Check sheet for the modelled part. Datum: model origin and axes. Units: mm. A direction names the side the tool comes from. Give positions to 0.01 mm unless a question says otherwise; leave off trailing zeros. Order: outer loops, then holes, each group sorted by start corner. A loop starts at its lowest first (then second) coordinate and runs counter-clockwise, first axis right, second up. Notation, with made-up numbers: (69, 36.5) -> (103, 36.5) arc R28 cw to (103, 59.5) -> close; hole circle Ø1 at (-8, 44). An arc over 180 degrees is marked (long way). One line per question, with ' | ' between items.
```python
from build123d import *

# Parameters (mm, degrees)
F1_DEPTH = 15
F3_DEPTH = 25
F4_R     = 3.99999
F5_W     = 7.0163438655
F5_H     = 17.1485144225
F6_DEPTH = 25
F7_R     = 2.6
F8_R     = 2.8
F9_DEPTH = 25
F10_R    = 20
F11_R    = 4


# Not quite as in the source:
# - a fillet or chamfer is up to 0.001 mm smaller than in the source, because OpenCascade refuses the exact size


with BuildPart() as f1:
    # F0 (on Right) → F1 (new body)
    with BuildSketch(Plane.YZ):
        Polygon((-44.9859467229, 8), (-66.9859467229, 8), (-66.9859467229, 0), (-44.9859467229, 0), (41.0894067598, -30.7737162478), (42.3002508738, -27.5966470596), (43.3758810707, -24.7743584453), (44.6834651639, -21.3434583933), align=None)
    extrude(amount=F1_DEPTH)

    # F2 (on face) → F3 (cut)
    with BuildSketch(Plane(origin=(0, 0, 0), x_dir=(1, 0, 0), z_dir=(0, 0, -1))):
        with BuildLine():
            Line((4.5, 58.9859467229), (4.5, 52.9859467229))
            ThreePointArc((4.5, 52.9859467229), (7.5, 49.9859467229), (10.5, 52.9859467229))
            Line((10.5, 52.9859467229), (10.5, 58.9859467229))
            ThreePointArc((10.5, 58.9859467229), (7.5, 61.9859467229), (4.5, 58.9859467229))
        make_face()
    extrude(amount=-F3_DEPTH, mode=Mode.SUBTRACT)

    # F4 (radius 4 in the source; OpenCascade refuses exactly that, so slightly less here)
    f4_edges = [f1.edges().sort_by_distance(p)[0] for p in [
        (7.5, -66.985947, 0),
        (7.5, -66.985947, 8),
    ]]
    fillet(f4_edges, radius=F4_R)

    # F5 (on face) → F6 (cut)
    with BuildSketch(Plane(origin=(0, -1.9867064016, -6.0710906068), x_dir=(1, 0, 0), z_dir=(0, 0.3110113487, 0.9504061979))):
        with Locations((11.4918280672, 40.5312428041)):
            Rectangle(F5_W, F5_H)
        Polygon((15, 49.1055000154), (15, 31.9569855928), (21.9836561345, 31.9569855928), (21.9836561345, 65.9569855928), (7.9836561345, 65.9569855928), (7.9836561345, 49.1055000154), align=None)
    extrude(amount=-F6_DEPTH, mode=Mode.SUBTRACT)

    # F7
    f7_edges = [f1.edges().sort_by_distance(p)[0] for p in [
        (7.983656, 26.888111, -20.58561),
        (15, 26.888111, -20.58561),
    ]]
    fillet(f7_edges, radius=F7_R)

    # F8 (on face) → F9 (cut)
    with BuildSketch(Plane.YZ.offset(15)):
        with Locations((37.2460966017, -24.0897076146)):
            Circle(F8_R)
    extrude(amount=-F9_DEPTH, mode=Mode.SUBTRACT)

    # F10
    f10_edges = [f1.edges().sort_by_distance(p)[0] for p in [
        (7.5, -44.985947, 8),
        (7.5, -44.985947, 0),
    ]]
    fillet(f10_edges, radius=F10_R)

    # F11
    f11_edges = [f1.edges().sort_by_distance(p)[0] for p in [
        (3.991828, 41.089407, -30.773716),
        (3.991828, 44.683465, -21.343458),
    ]]
    fillet(f11_edges, radius=F11_R)


solid = f1.part
```
Q1. Thickness scan on line 1 (Z direction, x = 11.5, y = -55.5); line 2 (X direction, y = 29.5, z = -26); line 3 (Z direction, x = 2.75, y = -29.5). Record the ranges inside material, lowest first.
Result sheet:
line 1: z = 0 to 8 | line 2: x = 0 to 7.98 | line 3: z = -5.54 to 2.93
Q2. Access from +Z, -Z, +X, -X, +Y, -Y to the whole of each face (thin tool, end or side, straight path). Record for faces 5 (the face through (7.6, -65.78, 6.86)), 6 (the face through (7.984, 34, -24)), 7 (the face through (7.566, -61.985, 3.944)).
Result sheet:
face 5: +Z, +X, -X, -Y | face 6: -Z, +X, +Y | face 7: +Z, -Z
Q3. Section check A-A (z = 5). Enter the section's corners in (x, y), and give its area (3 significant figures).
Result sheet:
outline: (0, -66.86) -> (15, -66.86) -> (15, -35.82) -> (0, -35.82) -> close; hole (4.5, -58.99) arc R3 ccw to (10.5, -58.99) -> (10.5, -52.99) arc R3 ccw to (4.5, -52.99) -> close | area: 401 mm2
Q4. Depth check by flat-ended pin: pin 1 Ø1.5 at (x, y) = (4.5, 9) entering from -Z; pin 2 Ø2 at (x, y) = (4.5, -42) entering from +Z; pin 3 Ø5 at (y, z) = (20.5, -8.5) entering from +X; pin 4 Ø8 at (x, y) = (10, 28.5) entering from +Z. Enter the tip coordinate at first touch or a pass-through.
Result sheet:
pin 1: stops at z = -19.57 | pin 2: stops at z = 7.32 | pin 3: passes through | pin 4: stops at z = -14.74
Q5. Mould release check, pull along Y, two halves, no side actions. Record for faces 1 (the face through (4, -56, 0)), 2 (the face through (4.5, -56, 4)), 3 (the face through (7.395, -2.714, -15.113)), 4 (the face through (4.048, 43.042, -22.077)): pulls with the +Y half, pulls with the -Y half, needs draft (parallel to the pull), parting line crosses it, or undercut.
Result sheet:
face 1: needs draft | face 2: undercut | face 3: pulls with the -Y half | face 4: pulls with the +Y half
Q6. Section check C-C (y = -13). Enter the section's corners in (x, z).
Result sheet:
outline: (0, -11.44) -> (15, -11.44) -> (15, -2.47) -> (0, -2.47) -> close
Q7. Section check D-D (z = -11.5). Enter the section's corners in (x, y), and give its area (3 significant figures).
Result sheet:
outline: (0, -12.82) -> (15, -12.82) -> (15, 14.6) -> (0, 14.6) -> close | area: 411 mm2
